from build123d import *

# Parameters (mm, degrees)
SKETCH1_W           = 250
SKETCH1_H           = 25
BOSS_EXTRUDE3_DEPTH = 20
SKETCH4_R           = 10
CUT_EXTRUDE3_DEPTH  = 20
SKETCH6_W           = 200
SKETCH6_H           = 20
BOSS_EXTRUDE4_DEPTH = 12.5
SKETCH7_W           = 200
SKETCH7_H           = 20
BOSS_EXTRUDE5_DEPTH = 12.5
CUT_EXTRUDE8_DEPTH  = 137.106575888
FILLET10_R          = 20
FILLET11_R          = 20
FILLET12_R          = 10
FILLET13_R          = 50
FILLET15_R          = 1


with BuildPart() as part:
    # Sketch1 → Boss-Extrude3 (new body)
    with BuildSketch(Plane.XY):
        Rectangle(SKETCH1_W, SKETCH1_H)
    extrude(amount=BOSS_EXTRUDE3_DEPTH)

    # Sketch4 → Cut-Extrude3 (cut)
    with BuildSketch(Plane.XY.offset(20)):
        with Locations((75, 0)):
            Circle(SKETCH4_R)
    extrude(amount=-CUT_EXTRUDE3_DEPTH, mode=Mode.SUBTRACT)

    # Sketch6 → Boss-Extrude4 (add)
    with BuildSketch(Plane(origin=(0, 12.5, 0), x_dir=(1, 0, 0), z_dir=(0, 1, 0))):
        with Locations((-25, -10)):
            Rectangle(SKETCH6_W, SKETCH6_H)
    extrude(amount=BOSS_EXTRUDE4_DEPTH)

    # Sketch7 → Boss-Extrude5 (add)
    with BuildSketch(Plane.XZ.offset(12.5)):
        with Locations((-25, 10)):
            Rectangle(SKETCH7_W, SKETCH7_H)
    extrude(amount=BOSS_EXTRUDE5_DEPTH)

    # Sketch8 → Cut-Extrude8 (cut, through all)
    with BuildSketch(Plane(origin=(0, 25, 0), x_dir=(1, 0, 0), z_dir=(0, 1, 0))):
        Polygon((-85, 0), (-125, 0), (-125, -10), (-105, -10), align=None)
    extrude(amount=-CUT_EXTRUDE8_DEPTH, mode=Mode.SUBTRACT)

    # Fillet10
    # the kernel refuses this fillet: 20 mm, written as the material it takes off along each edge
    with BuildSketch(Plane(origin=(-125, 68.301270189, 20), x_dir=(1, 0, 0), z_dir=(0, -1, 0))) as fillet10_piece_1:
        with BuildLine():
            CenterArc((17.320508076, -20), FILLET10_R, 90, 60)
            Line((0, -10), (-0.346410162, -9.8))
            ThreePointArc((-0.346410162, -9.8), (-0.4, -5), (-0.4, 0))
            Line((-0.4, 0), (0, 0.4))
            Line((0, 0.4), (17.320508076, 0.4))
            Line((17.320508076, 0.4), (17.320508076, 0))
        make_face()
    extrude(amount=136.602540378, mode=Mode.SUBTRACT)

    # Fillet11
    # the kernel refuses this fillet: 20 mm, written as the material it takes off along each edge
    with BuildSketch(Plane(origin=(75, -25, 66.351240544), x_dir=(-1, 0, 0), z_dir=(0, 0, -1))) as fillet11_piece_1:
        with BuildLine():
            CenterArc((18.540496218, 20), FILLET11_R, 202.024312837, 67.975687163)
            Line((0, 12.5), (-0.370809924, 12.35))
            ThreePointArc((-0.370809924, 12.35), (-0.4, 6.25), (-0.4, 0))
            Line((-0.4, 0), (0, -0.4))
            Line((0, -0.4), (18.540496218, -0.4))
            Line((18.540496218, -0.4), (18.540496218, 0))
        make_face()
    extrude(amount=112.702481089, mode=Mode.SUBTRACT)
    with BuildSketch(Plane(origin=(75, 25, -46.351240544), x_dir=(0, -1, 0), z_dir=(0, 0, 1))) as fillet11_piece_2:
        with BuildLine():
            CenterArc((20, -18.540496218), FILLET11_R, 112.024312837, 67.975687163)
            Line((0, -18.540496218), (-0.4, -18.540496218))
            Line((-0.4, -18.540496218), (-0.4, 0))
            Line((-0.4, 0), (0, 0.4))
            ThreePointArc((0, 0.4), (6.25, 0.4), (12.35, 0.370809924))
            Line((12.35, 0.370809924), (12.5, 0))
        make_face()
    extrude(amount=112.702481089, mode=Mode.SUBTRACT)

    # Fillet12
    fillet12_edges = [part.edges().sort_by_distance(p)[0] for p in [
        (125, -12.5, 10),
        (125, 12.5, 10),
    ]]
    fillet(fillet12_edges, radius=FILLET12_R)

    # Fillet13
    fillet13_edges = [part.edges().sort_by_distance(p)[0] for p in [
        (-85, 0, 0),
    ]]
    fillet(fillet13_edges, radius=FILLET13_R)

    # Fillet15
    fillet15_edges = [part.edges().sort_by_distance(p)[0] for p in [
        (65, 0, 20),
        (95, -12.5, 20),
        (-25.609994071, 25, 20),
        (-117.679491924, -25, 17.320508076),
        (-117.679491924, 25, 17.320508076),
        (-25.609994071, -25, 20),
        (67.63984367, 21.583123952, 20),
        (67.63984367, -21.583123952, 20),
        (95, 12.5, 20),
        (125, 0, 20),
        (122.071067812, -9.571067812, 20),
        (122.071067812, 9.571067812, 20),
    ]]
    fillet(fillet15_edges, radius=FILLET15_R)


solid = part.part
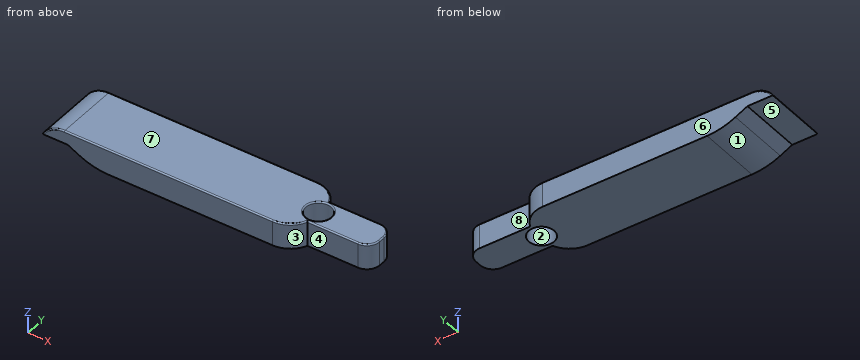
Here's how the part is built. I have some questions about the finished solid (model axes, mm). Face numbers are marked on the shaded views. A direction names the side the tool comes from. Give positions to 0.01 mm unless a question says otherwise; leave off trailing zeros. Write each loop counter-clockwise with the first axis right and the second up, starting at its lowest first coordinate (ties: lowest second). Pieces come first, ordered by that corner, then holes. Notation, with made-up numbers: (-26, -22) -> (-22, -22) arc R25 ccw to (-22, -10) -> close; hole circle Ø9 at (-40, 76.25). An arc over 180 degrees is marked (long way). Use one line per item in the form item = value. Start each with the question number.
1. Imagine slicing it at A-A on y = 0. List the corners of the cut face in (x, z) for me.
2. If I drill on L1, parallel to Y at x = 75, z = 15; L2, parallel to Z at x = -108, y = -21.5; L3, parallel to X at y = -1, z = 15.5, over which ranges is the centre line in solid material (lowest first)?
3. Imagine slicing it at C-C on x = -81. List the corners of the cut face in (y, z) for me, plus the area to 3 significant figures.
4. On a 3-axis mill with a long thin cutter (end or side, diameter ignored), from which of +Z, -Z, +X, -X, +Y, -Y can I reach the whole of each face in a straight line? I mean the marked faces 4, 5, 6, 7 and 8. Say none if no direction works.
5. Will these pins go through, and if not, where does the flat tip stop? pin 1 Ø2 at (y, z) = (0, 3.5) entering from -X; pin 2 Ø1.5 at (x, y) = (-98, 3.5) entering from -Z (3 decimals); pin 3 Ø8 at (y, z) = (12, 2) entering from -X.
6. Thinking about a two-plate mould opening in Y: for the marked faces 1, 2 and 3, which applies, +Y half, -Y half, draft (parallel to the pull), parting line (faces both ways), or undercut?
7. Imagine slicing it at B-B on x = 101. List the corners of the cut face in (y, z) for me, plus the area to 3 significant figures.
Entries:
q1.outline = (-125, 10) -> (-105, 10) -> (-95.56, 5.28) arc R50 ccw to (-73.2, 0) -> (65, 0) -> (65, 19) arc R1 ccw to (64, 20) -> (-107.68, 20) arc R20 ccw to start; (85, 0) -> (125, 0) -> (125, 19) arc R1 ccw to (124, 20) -> (86, 20) arc R1 ccw to (85, 19) -> close
q2.L1 = -12.5 to -10, 10 to 12.5
q2.L2 = 10 to 20
q2.L3 = -120.32 to 65.05, 84.95 to 125
q3.outline = (-25, 0.61) -> (25, 0.61) -> (25, 19) arc R1 ccw to (24, 20) -> (-24, 20) arc R1 ccw to (-25, 19) -> close
q3.area = 969 mm²
q4.face_4 = +Z, -Z, +X, -Y
q4.face_5 = -Z, -X, +Y, -Y
q4.face_6 = +Z, -Z, +X, -X, +Y
q4.face_7 = +Z, +X, -X, +Y, -Y
q4.face_8 = +Z, -Z, +X, +Y
q5.pin_1 = -93.93
q5.pin_2 = 6.125
q5.pin_3 = -97
q6.face_1 = draft
q6.face_2 = undercut
q6.face_3 = -Y half
q7.outline = (-12.5, 0) -> (12.5, 0) -> (12.5, 19) arc R1 ccw to (11.5, 20) -> (-11.5, 20) arc R1 ccw to (-12.5, 19) -> close
q7.area = 500 mm²
